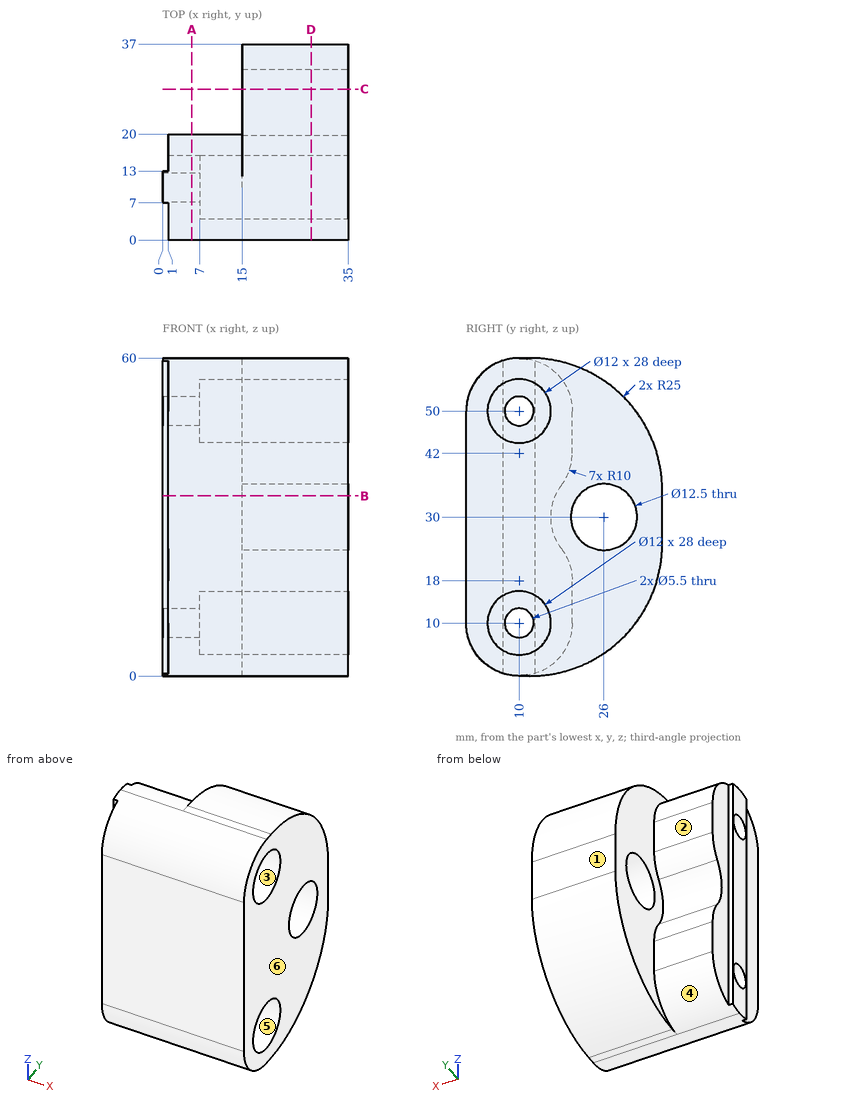
Source: three-view drawing plus pictorial views. Frame: mm from the lowest corner of the part. A direction names the side the tool comes from. Round coordinates to 2 decimals unless told otherwise and drop trailing zeros. Loops run counter-clockwise (first coordinate to the right, second up) from the corner with the lowest first, then second, coordinate; pieces in that order, holes last. Notation, with made-up numbers: (-24, 75.5) - (33, 75.5) arc R21 cw to (33, 100.5) - close; hole circle Ø1 at (25.5, 88.5). An arc over 180 degrees is marked (long way). Write item = value, one per line. Start each with the question number.
Item 1: First-contact query: pin 1 Ø5.5 at (y, z) = (17, 32.5) entering from -X; pin 2 Ø0.8 at (x, z) = (0.5, 25) entering from +Y; pin 3 Ø12 at (x, z) = (26, 39.5) entering from +Y; pin 4 Ø10 at (x, z) = (21, 43) entering from +Y. Flat tips, straight axial feed; report the tip coordinate or a pass-through.
Item 2: Section query D-D on x = 28. Output: boundary loops of the cut face in (y, z), plus the area to 3 significant figures.
Item 3: Section query B-B on z = 34. Output: boundary loops of the cut face in (x, y) (1 decimal).
Item 4: Section query C-C on y = 28.5. Output: boundary loops of the cut face in (x, z), plus the area to 3 significant figures.
Item 5: Mould query, pull axis Z, two halves, no side actions, for the marked faces 4, 5 and 6. Classes: released by +Z, released by -Z, zero draft, split by the parting line, or undercut.
Item 6: Section query A-A on x = 5.5. Count the separate pieces of the cut face and the enclosed holes in it, plus the area to 3 significant figures.
Item 7: Reachability of the marked faces 1, 2 and 3 from +Z, -Z, +X, -X, +Y, -Y: full face, straight path, thin tool, end or side. Return the list, or none.
Item 8: Material intervals for line 1 (Z direction, x = 28.5, y = 9.5); line 2 (Z direction, x = 25, y = 11); line 3 (Y direction, x = 2, z = 50), sorted ascending.
Results list:
q1.pin_1 = 1
q1.pin_2 = 13
q1.pin_3 = 37
q1.pin_4 = 36.82
q2.outline = (0, 10) arc R10 ccw to (10, 0) - (12, 0) arc R25 ccw to (37, 25) - (37, 35) arc R25 ccw to (12, 60) - (10, 60) arc R10 ccw to (0, 50) - close; hole circle Ø12 at (10, 10); hole circle Ø12 at (10, 50); hole circle Ø12.5 at (26, 30)
q2.area = 1,560 mm²
q3.outline = (0, 7) - (1, 7) - (1, 0) - (35, 0) - (35, 21.2) - (15, 21.2) - (15, 16.8) - (1, 16.8) - (1, 13) - (0, 13) - close; (15, 30.8) - (35, 30.8) - (35, 37) - (15, 37) - close
q4.outline = (15, 6.22) - (35, 6.22) - (35, 24.27) - (15, 24.27) - close; (15, 35.73) - (35, 35.73) - (35, 53.78) - (15, 53.78) - close
q4.area = 722 mm²
q5.face_4 = released by -Z
q5.face_5 = undercut
q5.face_6 = zero draft
q6.separate_pieces = 1
q6.enclosed_holes = 2
q6.area = 1,020 mm²
q7.face_1 = +Z, -Z, +X, -X, +Y
q7.face_2 = +Z, -Z, -X, +Y
q7.face_3 = +X
q8.line_1 = 0.01 to 4.02, 15.98 to 44.02, 55.98 to 59.99
q8.line_2 = 0 to 4.08, 15.92 to 44.08, 55.92 to 60
q8.line_3 = 0 to 7.25, 12.75 to 20
